The model under review builds one solid part; all positions refer to its coordinate system, in mm. Face numbers are marked on the shaded views. A direction names the side the tool comes from. Coordinates: 2 decimals unless noted, no trailing zeros. Order: outer loops, then holes, each group sorted by start corner. A loop starts at its lowest first (then second) coordinate and runs counter-clockwise, first axis right, second up. Notation, with made-up numbers: (6.25, 63.5) -> (17.25, 63.5) arc R23 cw to (17.25, 98.5) -> close; hole circle Ø2 at (-27, 54.25). An arc over 180 degrees is marked (long way). Use one line per item in the form item = value. Start each with the question number.
(1) Take a section at D-D (z = 71). State the section outline as (x, y) points.
(2) Take a section at C-C (z = 104). State the section outline as (x, y) points.
(3) Take a section at B-B (x = 52). State the section outline as (y, z) points.
(4) For the marked faces 4, 5, 6 and 7, list the 3-axis set-ups (+Z, -Z, +X, -X, +Y, -Y) from which the entire face can be reached by the end or side of a thin tool; tool diameter is ignored.
(5) Insertion check: pin 1 Ø12 at (x, y) = (113, 10.5) entering from +Z; pin 2 Ø2 at (x, y) = (-112.5, 18) entering from +Z; pin 3 Ø10 at (y, z) = (4.5, -33.5) entering from +X; pin 4 Ø12 at (x, z) = (-82, 88) entering from -Y. Each pin has a flat end and moves straight along its axis. Give the tip position at first contact, or say it passes through.
(6) Take a section at A-A (z = -41.5). State the section outline as (x, y) points, then the cut area to 3 significant figures.
(7) Wall thickness on line 1 along Z through (x, y) = (-123.5, -15); line 2 along Z through (x, y) = (130, -17.5); line 3 along Z through (x, y) = (-87.5, 23): over which ranges is each line inside the solid? List them lowest first.
(8) Mouldability with a two-part tool opening along Z and no side actions: class the marked faces 1, 2 and 3 as +Z half, -Z half, draft (parallel to the pull), parting line (faces both ways), or undercut.
```python
from build123d import *

# Parameters (mm, degrees)
BOSS_EXTRUDE1_DEPTH        = 62.5
BOSS_EXTRUDE1_DEPTH_BACK   = 62.5
SKETCH2_R                  = 20
BOSS_EXTRUDE1_2_DEPTH      = 62.5
BOSS_EXTRUDE1_2_DEPTH_BACK = 62.5
SKETCH4_R                  = 5
BOSS_EXTRUDE5_DEPTH        = 5
SKETCH9_R                  = 5
BOSS_EXTRUDE6_DEPTH        = 25
BOSS_EXTRUDE8_OUTLINE_R    = 5
BOSS_EXTRUDE8_DEPTH        = 10
SKETCH12_W                 = 200
SKETCH12_H                 = 10
BOSS_EXTRUDE9_DEPTH        = 135
SKETCH15_R                 = 5
BOSS_EXTRUDE10_DEPTH       = 6
SKETCH16_R                 = 20
BOSS_EXTRUDE11_DEPTH       = 50
MIRROR6_COPY_1_SKETCH_R    = 5
MIRROR6_COPY_1_DEPTH       = 25
MIRROR6_COPY_2_SKETCH_R    = 5
MIRROR6_COPY_2_DEPTH       = 25
SKETCH17_R                 = 2.5
BOSS_EXTRUDE12_DEPTH       = 2
BOSS_EXTRUDE13_START       = 6
SKETCH18_R                 = 5
BOSS_EXTRUDE13_DEPTH       = 6
SKETCH20_R                 = 1
BOSS_EXTRUDE15_DEPTH       = 1


# Read off the part's stored shape, not the designer's step: Boss-Extrude8
with BuildPart() as part:
    # Sketch2 → Boss-Extrude1 (new, two sides: drawn at the far end of the back side and taken through both)
    with BuildSketch(Plane.XY.offset(-BOSS_EXTRUDE1_DEPTH_BACK)):
        with Locations((-130, 0)):
            Circle(SKETCH2_R)
    extrude(amount=BOSS_EXTRUDE1_DEPTH + BOSS_EXTRUDE1_DEPTH_BACK)

    # Sketch4 → Boss-Extrude5 (add)
    with BuildSketch(Plane.XY.offset(62.5)):
        with Locations((-130, 0)):
            Circle(SKETCH4_R)
    boss_extrude5 = extrude(amount=BOSS_EXTRUDE5_DEPTH)

    # Mirror2: Boss-Extrude5 across plane
    add(boss_extrude5.mirror(Plane.XY))



with BuildPart() as body_2:
    # Sketch2 → Boss-Extrude1 2 (new, two sides: drawn at the far end of the back side and taken through both)
    with BuildSketch(Plane.XY.offset(-BOSS_EXTRUDE1_2_DEPTH_BACK)):
        with Locations((130, 0)):
            Circle(SKETCH2_R)
    extrude(amount=BOSS_EXTRUDE1_2_DEPTH + BOSS_EXTRUDE1_2_DEPTH_BACK)

    # Sketch9 → Boss-Extrude6 (add)
    with BuildSketch(Plane.XY.offset(62.5)):
        with Locations((130, 0)):
            Circle(SKETCH9_R)
    boss_extrude6 = extrude(amount=BOSS_EXTRUDE6_DEPTH)

    # Mirror4: Boss-Extrude6 across plane
    add(boss_extrude6.mirror(Plane.XY))


with BuildPart() as part_1:
    add(part.part)

    add(body_2.part)  # Boss-Extrude8 merges body 2
    # Boss-Extrude8 outline → Boss-Extrude8 (add)
    with BuildSketch(Plane.XY.offset(67.5)):
        with BuildLine():
            ThreePointArc((130, -30), (160, 0), (130, 30))
            Line((130, 30), (-130, 30))
            ThreePointArc((-130, 30), (-160, 0), (-130, -30))
            Line((-130, -30), (130, -30))
        make_face()
        with Locations((130, 0)):
            Circle(BOSS_EXTRUDE8_OUTLINE_R, mode=Mode.SUBTRACT)
    boss_extrude8 = extrude(amount=BOSS_EXTRUDE8_DEPTH)

    # Mirror5: Boss-Extrude8 across plane
    add(boss_extrude8.mirror(Plane.XY))

    # Sketch12 → Boss-Extrude9 (add)
    with BuildSketch(Plane.XY.offset(-67.5)):
        Rectangle(SKETCH12_W, SKETCH12_H)
    extrude(amount=BOSS_EXTRUDE9_DEPTH)

    # Sketch15 → Boss-Extrude10 (add)
    with BuildSketch(Plane.XY.offset(77.5)):
        with Locations((-130, 0)):
            Circle(SKETCH15_R)
    extrude(amount=BOSS_EXTRUDE10_DEPTH)

    # Sketch16 → Boss-Extrude11 (add)
    with BuildSketch(Plane.XY.offset(83.5)):
        with Locations((-130, 0)):
            Circle(SKETCH16_R)
    extrude(amount=BOSS_EXTRUDE11_DEPTH)

    # Mirror6 copy 1 sketch → Mirror6 copy 1 (add)
    with BuildSketch(Plane(origin=(0, 0, -62.5), x_dir=(-1, 0, 0), z_dir=(0, 0, -1))):
        with Locations((130, 0)):
            Circle(MIRROR6_COPY_1_SKETCH_R)
    extrude(amount=MIRROR6_COPY_1_DEPTH)

    # Mirror6 copy 2 sketch → Mirror6 copy 2 (add)
    with BuildSketch(Plane(origin=(0, 0, 62.5), x_dir=(-1, 0, 0), z_dir=(0, 0, 1))):
        with Locations((130, 0)):
            Circle(MIRROR6_COPY_2_SKETCH_R)
    extrude(amount=MIRROR6_COPY_2_DEPTH)

    # Sketch17 → Boss-Extrude12 (add)
    with BuildSketch(Plane.XY.offset(133.5)):
        with Locations((-139.88898439, 0)):
            Circle(SKETCH17_R)
        with Locations((-120.11101561, 0)):
            Circle(SKETCH17_R)
    extrude(amount=BOSS_EXTRUDE12_DEPTH)

    # Sketch18 → Boss-Extrude13 (add)
    with BuildSketch(Plane.XY.offset(77.5).offset(BOSS_EXTRUDE13_START)):
        with BuildLine():
            Line((-133.842725931, 6.440765282), (-146.688296152, 18.721665833))
            ThreePointArc((-146.688296152, 18.721665833), (-149.516009312, 18.658118354), (-149.452461834, 15.830405194))
            Line((-149.452461834, 15.830405194), (-136.606891613, 3.549504643))
            ThreePointArc((-136.606891613, 3.549504643), (-137.498106816, -0.168505698), (-136.440765282, -3.842725931))
            Line((-136.440765282, -3.842725931), (-148.721665833, -16.688296152))
            ThreePointArc((-148.721665833, -16.688296152), (-148.658118354, -19.516009312), (-145.830405194, -19.452461834))
            Line((-145.830405194, -19.452461834), (-133.549504643, -6.606891613))
            ThreePointArc((-133.549504643, -6.606891613), (-129.831494302, -7.498106816), (-126.157274069, -6.440765282))
            Line((-126.157274069, -6.440765282), (-113.311703848, -18.721665833))
            ThreePointArc((-113.311703848, -18.721665833), (-110.483990688, -18.658118354), (-110.547538166, -15.830405194))
            Line((-110.547538166, -15.830405194), (-123.393108387, -3.549504643))
            ThreePointArc((-123.393108387, -3.549504643), (-122.501893184, 0.168505698), (-123.559234718, 3.842725931))
            Line((-123.559234718, 3.842725931), (-111.278334167, 16.688296152))
            ThreePointArc((-111.278334167, 16.688296152), (-111.341881646, 19.516009312), (-114.169594806, 19.452461834))
            Line((-114.169594806, 19.452461834), (-126.450495357, 6.606891613))
            ThreePointArc((-126.450495357, 6.606891613), (-130.168505698, 7.498106816), (-133.842725931, 6.440765282))
        make_face()
        with Locations((-130, 0)):
            Circle(SKETCH18_R, mode=Mode.SUBTRACT)
    extrude(amount=-BOSS_EXTRUDE13_DEPTH)

    # Sketch20 → Boss-Extrude15 (add)
    with BuildSketch(Plane.XY.offset(83.5)):
        with Locations((-148.070378993, 17.276035513)):
            Circle(SKETCH20_R)
        with Locations((-112.723964487, 18.070378993)):
            Circle(SKETCH20_R)
        with Locations((-147.276035513, -18.070378993)):
            Circle(SKETCH20_R)
        with Locations((-111.929621007, -17.276035513)):
            Circle(SKETCH20_R)
    extrude(amount=BOSS_EXTRUDE15_DEPTH)


solid = part_1.part
```
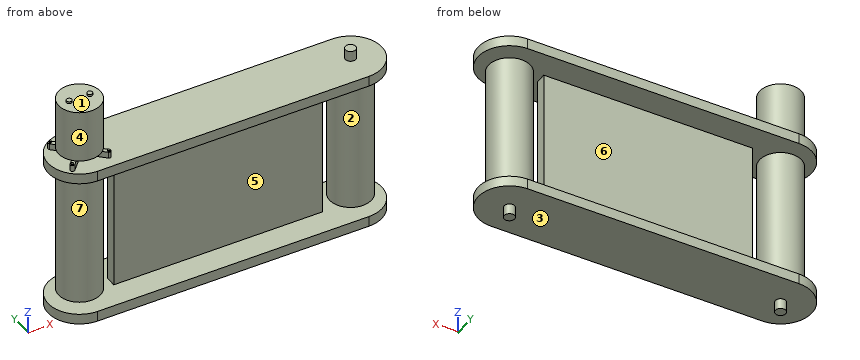
Findings:
q1.outline = (-130, -30) -> (130, -30) arc R30 ccw to (130, 30) -> (-130, 30) arc R30 ccw to start
q2.outline = circle Ø40 at (-130, 0)
q3.outline = (-30, -77.5) -> (30, -77.5) -> (30, -67.5) -> (5, -67.5) -> (5, 67.5) -> (30, 67.5) -> (30, 77.5) -> (-30, 77.5) -> (-30, 67.5) -> (-5, 67.5) -> (-5, -67.5) -> (-30, -67.5) -> close
q4.face_4 = +Z
q4.face_5 = -Y
q4.face_6 = +Y
q4.face_7 = none
q5.pin_1 = 77.5
q5.pin_2 = 84.5
q5.pin_3 = 150
q5.pin_4 = through
q6.outline = circle Ø40 at (-130, 0); (-100, -5) -> (100, -5) -> (100, 5) -> (-100, 5) -> close; circle Ø40 at (130, 0)
q6.area = 4,510 mm²
q7.line_1 = -77.5 to -67.5, -62.5 to 62.5, 67.5 to 77.5, 83.5 to 133.5
q7.line_2 = -77.5 to -67.5, -62.5 to 62.5, 67.5 to 77.5
q7.line_3 = -77.5 to -67.5, 67.5 to 77.5
q8.face_1 = +Z half
q8.face_2 = undercut
q8.face_3 = -Z half
